Autodesk Inventor part; units mm, degrees
ref_plane "YZ Plane" through (0, 0, 0) normal (1, 0, 0) x (0, 1, 0)
ref_plane "XZ Plane" through (0, 0, 0) normal (0, 1, 0) x (-1, 0, 0)
ref_plane "XY Plane" through (0, 0, 0) normal (0, 0, 1) x (1, 0, 0)
sketch "Sketch1" plane through (0, 0, 0) normal (0, 0, 1) x (1, 0, 0)
  line L0 (-42.5, -20) -> (42.5, -20)
  line L1 (42.5, -20) -> (42.5, 20)
  line L2 (42.5, 20) -> (-42.5, 20)
  line L3 (-42.5, 20) -> (-42.5, -20)
  line L4 (-42.5, -20) -> (42.5, 20) construction
  line L5 (42.5, -20) -> (-42.5, 20) construction
  point P0 (0, 0)
  dimension "d0" = 85
  dimension "d1" = 40
extrude "Extrusion1" add sketch "Sketch1" along normal blind 1
fillet "Fillet1" radius 3.175 4 edges at (-42.5, 0, 1) (0, 20, 1) (0, -20, 1) (42.5, 0, 1)
sketch "Sketch2" plane through (0, 0, 1) normal (0, 0, 1) x (1, 0, 0)
  line L0 (-40.187, -17.687) -> (-40.187, 17.687) construction
  line L1 (-40.187, 0) -> (40.187, 0) construction
  line L2 (40.187, 17.687) -> (40.187, -17.687) construction
  line L3 (-40.187, 17.687) -> (40.187, 17.687) construction
  line L4 (0, 17.687) -> (0, -17.687) construction
  line L5 (40.187, -17.687) -> (-40.187, -17.687) construction
  line L6 (10, -10) -> (-10, -10)
  line L7 (-10, -10) -> (-10, 10)
  line L8 (-10, 10) -> (10, 10)
  line L9 (10, 10) -> (10, -10)
  line L10 (10, -10) -> (-10, 10) construction
  line L11 (-10, -10) -> (10, 10) construction
  point P0 (0, 0)
  dimension "d5" = 20
  dimension "d6" = 20
extrude "Extrusion2" add sketch "Sketch2" along normal blind 25.4
sketch "Sketch3" plane through (-10, -10, 1) normal (0, -1, 0) x (1, 0, 0)
  line L0 (20, 25.4) -> (0, 25.4)
  line L1 (20, 0) -> (20, 25.4)
  line L2 (0, 25.4) -> (20, 25.4)
  line L3 (20, 25.4) -> (20, 15.1947)
  line L4 (20, 15.1947) -> (0, 15.1947)
  line L5 (0, 15.1947) -> (0, 25.4)
  point P0 (10, -1)
sketch "Sketch4" plane through (0, 0, 26.4) normal (0, 0, 1) x (1, 0, 0)
  line L0 (-10, -10) -> (-10, 10) construction
  line L1 (-10, 0) -> (10, 0) construction
  line L2 (10, 10) -> (10, -10) construction
  point P0 (0, 0)
ref_plane "Work Plane1" through (-10, 0, 26.4) normal (0, -1, 0) x (1, 0, 0)
extrude "Extrusion3" add sketch "Sketch3" along normal blind 25.4
mirror "Mirror1" about plane through (-10, 0, 26.4) normal (0, -1, 0) of "Extrusion3"
fillet "Fillet2" radius 5.08 2 edges at (0, -10, 16.1947) (0, 10, 16.1947)
fillet "Fillet3" radius 5.08 22 edges at (-10, 35.4, 21.2974) (10, 35.4, 21.2974) (0, 35.4, 16.1947) (0, 35.4, 26.4) (-10, 0, 26.4) (-10, -35.4, 21.2974) (10, -35.4, 21.2974) (10, 0, 26.4) (10, 11.4879, 14.7068) (10, 10, 6.0574) (10, 25.24, 16.1947) (-10, 11.4879, 14.7068) (-10, 10, 6.0574) (-10, 25.24, 16.1947) (-10, -11.4879, 14.7068) (-10, -10, 6.0574) (-10, -25.24, 16.1947) (0, -35.4, 16.1947) (10, -11.4879, 14.7068) (10, -10, 6.0574) (10, -25.24, 16.1947) (0, -35.4, 26.4)
sketch "Sketch5" plane through (0, 0, 1) normal (0, 0, 1) x (1, 0, 0)
  circle A0 centre (-35.8589, 13.4243) radius 2.8
  line L0 (59.5, 0) -> (-59.5, 0)
  line L1 (10, 4.92) -> (10, -4.92)
  arc A1 (4.92, -10) -> (10, -4.92) centre (4.92, -4.92) ccw
  line L2 (4.92, -10) -> (-4.92, -10)
  arc A2 (-10, -4.92) -> (-4.92, -10) centre (-4.92, -4.92) ccw
  line L3 (-10, -4.92) -> (-10, 4.92)
  arc A3 (-4.92, 10) -> (-10, 4.92) centre (-4.92, 4.92) ccw
  line L4 (-4.92, 10) -> (4.92, 10)
  arc A4 (10, 4.92) -> (4.92, 10) centre (4.92, 4.92) ccw
  line L5 (40.187, 17.687) -> (40.187, -17.687)
  line L6 (-40.187, 17.687) -> (40.187, 17.687)
  line L7 (-40.187, -17.687) -> (-40.187, 17.687)
  line L8 (40.187, -17.687) -> (-40.187, -17.687)
  circle A5 centre (-35.8589, -13.4243) radius 2.8
  line L9 (42.5, 20) -> (-42.5, 20) construction
  line L10 (0, 20) -> (0, -20) construction
  line L11 (-42.5, -20) -> (42.5, -20) construction
  circle A6 centre (35.8589, 13.4243) radius 2.8
  circle A7 centre (35.8589, -13.4243) radius 2.8
  point P0 (0, 0)
  dimension "d14" = 5.6
extrude "Extrusion4" cut sketch "Sketch5" against normal blind 345.1324 contours A0 | A5 | A6 | A7
chamfer "Chamfer1" distance 1 angle 45 4 edges at (33.0589, 13.4243, 1) (33.0589, -13.4243, 1) (-38.6589, 13.4243, 1) (-38.6589, -13.4243, 1)
properties part number "WireWrappoMatica(TM)"
Design review of the part built by this model. Coordinates are the model's own, in mm. A direction names the side the tool comes from. Give positions to 0.01 mm unless a question says otherwise; leave off trailing zeros. Loops run counter-clockwise (first coordinate to the right, second up) from the corner with the lowest first, then second, coordinate; pieces in that order, holes last. Notation, with made-up numbers: M 53.25,53.25 L 106.25,53.25 A15 ccw 106.25,75.25 Z; hole C -10.5,16 d10. An arc over 180 degrees is marked long. Write item = value, one per line.
Q1. We need section B-B (z = 8.75). Give the boundary of the cut face in (x, y), plus the area to 3 significant figures.
Output values:
outline = M -10,-4.92 A5.08 ccw -4.92,-10 L 4.92,-10 A5.08 ccw 10,-4.92 L 10,4.92 A5.08 ccw 4.92,10 L -4.92,10 A5.08 ccw -10,4.92 Z
area = 378 mm^2
Q2. We need section D-D (x = -22.5). Give the boundary of the cut face in (y, z) (3 decimals).
Output values:
outline = M -20,0 L 20,0 A3.175 ccw 17.687,1 L -17.687,1 A3.175 ccw Z
Q3. To check wall thickness, follow line 1 (Y direction, x = -0.5, z = 11); line 2 (Z direction, x = -2, y = 15.5). State the ranges of each line that lie inside material, in increasing order. Write a range as [from, to].
Output values:
line_1 = [-10, 10]
line_2 = [0, 1], [16.19, 26.4]
Q4. We need section A-A (y = -0.5). Give the boundary of the cut face in (x, z) (3 decimals), plus the area to 3 significant figures.
Output values:
outline = M -42.5,0 L 42.5,0 A3.175 ccw 40.187,1 L 10,1 L 10,21.32 A5.08 ccw 4.92,26.4 L -4.92,26.4 A5.08 ccw -10,21.32 L -10,1 L -40.187,1 A3.175 ccw Z
area = 580 mm^2
Q5. We need section C-C (x = 36). Count the separate pieces of the cut face and the enclosed holes in it, plus the area to 3 significant figures.
Output values:
separate_pieces = 3
enclosed_holes = 0
area = 25.4 mm^2
Q6. Draft analysis for pull direction Z (two halves, no side actions). For faces 6 (the cylindrical face through (-8.55, 22.59, 17.72)), 7 (the flat face through (0, 0, 26.4)), 8 (the flat face through (10, 0, 13)), state which applies: +Z half, -Z half, draft (parallel to the pull), parting line (faces both ways), or undercut.
Output values:
face_6 = undercut
face_7 = +Z half
face_8 = draft
Q7. For faces 1 (the cylindrical face through (8.472, 8.551, 5.987)), 2 (the flat face through (0, -10, 6)), 3 (the cylindrical face through (-8.472, -8.551, 5.987)), 4 (the cylindrical face through (0.595, 18.964, 0.732)), 5 (the cylindrical face through (8.55, -22.59, 17.72)), list the 3-axis set-ups (+Z, -Z, +X, -X, +Y, -Y) from which the entire face can be reached by the end or side of a thin tool; tool diameter is ignored.
Output values:
face_1 = +X, +Y
face_2 = +X, -X, -Y
face_3 = -X, -Y
face_4 = +X, -X, +Y
face_5 = +X, -Y
Q8. Insertion check: pin 1 (10 mm diameter, centred on x = 7, z = 11, fed in from -Y); pin 2 (11 mm diameter, centred on x = -1.5, z = 7.5, fed in from -Y); pin 3 (2 mm diameter, centred on x = -8.5, z = 19.5, fed in from +Y). Each pin has a flat end and moves straight along its axis. Give the tip position at first contact, or say it passes through.
Output values:
pin_1 = -13.06
pin_2 = -10.36
pin_3 = 34.42
